Read the model definition and answer for the solid it produces. Units are mm, in the model's axes. Face numbers are marked on the shaded views. A direction names the side the tool comes from. Round coordinates to 2 decimals unless told otherwise and drop trailing zeros. Order: outer loops, then holes, each group sorted by start corner. A loop starts at its lowest first (then second) coordinate and runs counter-clockwise, first axis right, second up. Notation, with made-up numbers: (-16, -2) - (30, -2) arc R22 cw to (30, 5) - close; hole circle Ø4 at (7.25, 9). An arc over 180 degrees is marked (long way). Answer as a JSON object with one key per item and string values. Group by question number.
Q1. Given pin 1 Ø5 at (x, z) = (25.5, 93) entering from +Y; pin 2 Ø7.5 at (y, z) = (-12.5, 79) entering from -X; pin 3 Ø5.5 at (x, y) = (20, 34) entering from +Z; pin 4 Ø6.5 at (x, y) = (0, 17.5) entering from -Z (3 decimals), each flat-ended and moving along its own axis, determine where each tip first touches the part or whether it passes through.
Q2. Consider line 1 (Y direction, x = 0, z = -1); line 2 (Y direction, x = 0, z = 2); line 3 (Y direction, x = 20, z = 2). Determine where each line is inside the solid, lowest interval first.
Q3. A cutting plane is placed at A-A on y = -12.5. Count the separate pieces of the cut face and the enclosed holes in it, and give its area (3 significant figures).
Q4. A tool of negligible diameter and unlimited length cuts with its end or side. For the marked faces 5, 6, 7, 8 and 9, from which of +Z, -Z, +X, -X, +Y, -Y can it reach the whole face along a straight path? Write none if from no direction.
Q5. A cutting plane is placed at C-C on y = 32.5. Determine the outline of the cut face in (x, z).
Q6. The mould has two halves that part along X. Classify the marked faces 1, 2, 3 and 4: pulls with the +X half, pulls with the -X half, needs draft (parallel to the pull), parting line crosses it, or undercut.
Q7. A cutting plane is placed at B-B on x = -49. Determine the outline of the cut face in (y, z).
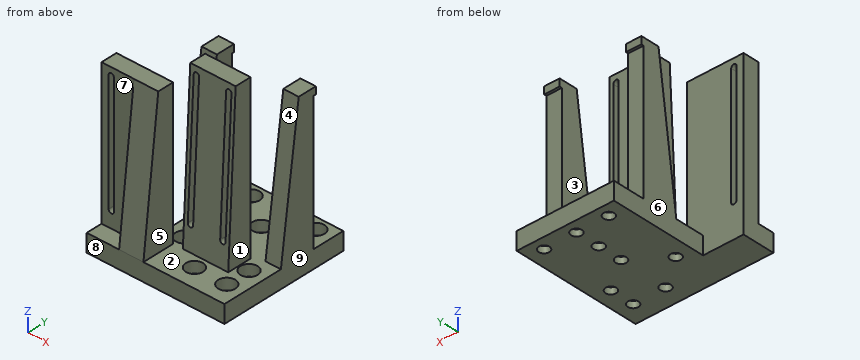
```python
from build123d import *

# Parameters (mm, degrees)
SKETCH1_W                 = 60
SKETCH1_H                 = 80
SKETCH1_R                 = 3.3
BOSS_EXTRUDE1_DEPTH       = 4
SKETCH3_W                 = 60
SKETCH3_H                 = 80
SKETCH3_R                 = 5.3
BOSS_EXTRUDE2_DEPTH       = 7
SKETCH4_W                 = 9.5
SKETCH4_H                 = 10
BOSS_EXTRUDE3_DEPTH       = 89
BOSS_EXTRUDE4_DEPTH       = 9.5
BOSS_EXTRUDE5_DEPTH       = 9.5
SKETCH7_W                 = 9.5
SKETCH7_H                 = 4.5
BOSS_EXTRUDE6_DEPTH       = 1.5
SKETCH9_W                 = 28
SKETCH9_H                 = 10
BOSS_EXTRUDE7_DEPTH       = 100
BOSS_EXTRUDE9_DEPTH       = 28
CUT_EXTRUDE1_DEPTH        = 18
BOSS_EXTRUDE10_DEPTH      = 25
BOSS_EXTRUDE10_DEPTH_BACK = 10
SKETCH13_W                = 100
SKETCH13_H                = 10
SKETCH14_W                = 11
SKETCH14_H                = 20
BOSS_EXTRUDE11_DEPTH      = 25
CUT_EXTRUDE2_DEPTH        = 10
BOSS_EXTRUDE12_DEPTH      = 15


with BuildPart() as part:
    # Sketch1 → Boss-Extrude1 (new body)
    with BuildSketch(Plane.XY):
        Rectangle(SKETCH1_W, SKETCH1_H)
        with Locations((-20, -12.5)):
            Circle(SKETCH1_R, mode=Mode.SUBTRACT)
        with Locations((20, -12.5)):
            Circle(SKETCH1_R, mode=Mode.SUBTRACT)
        with Locations((0, 17.5)):
            Circle(SKETCH1_R, mode=Mode.SUBTRACT)
        with Locations((0, 2.5)):
            Circle(SKETCH1_R, mode=Mode.SUBTRACT)
        with Locations((20, 32.5)):
            Circle(SKETCH1_R, mode=Mode.SUBTRACT)
        with Locations((0, 32.5)):
            Circle(SKETCH1_R, mode=Mode.SUBTRACT)
        with Locations((-20, 32.5)):
            Circle(SKETCH1_R, mode=Mode.SUBTRACT)
        with Locations((0, -27.5)):
            Circle(SKETCH1_R, mode=Mode.SUBTRACT)
        with Locations((20, -27.5)):
            Circle(SKETCH1_R, mode=Mode.SUBTRACT)
    extrude(amount=-BOSS_EXTRUDE1_DEPTH)

    # Sketch3 → Boss-Extrude2 (add)
    with BuildSketch(Plane.XY):
        Rectangle(SKETCH3_W, SKETCH3_H)
        with Locations((0, 17.5)):
            Circle(SKETCH3_R, mode=Mode.SUBTRACT)
        with Locations((-20, -12.5)):
            Circle(SKETCH3_R, mode=Mode.SUBTRACT)
        with Locations((20, -12.5)):
            Circle(SKETCH3_R, mode=Mode.SUBTRACT)
        with Locations((0, 2.5)):
            Circle(SKETCH3_R, mode=Mode.SUBTRACT)
        with Locations((-20, 32.5)):
            Circle(SKETCH3_R, mode=Mode.SUBTRACT)
        with Locations((0, 32.5)):
            Circle(SKETCH3_R, mode=Mode.SUBTRACT)
        with Locations((20, 32.5)):
            Circle(SKETCH3_R, mode=Mode.SUBTRACT)
        with Locations((0, -27.5)):
            Circle(SKETCH3_R, mode=Mode.SUBTRACT)
        with Locations((20, -27.5)):
            Circle(SKETCH3_R, mode=Mode.SUBTRACT)
    extrude(amount=BOSS_EXTRUDE2_DEPTH)

    # Sketch4 → Boss-Extrude3 (add)
    with BuildSketch(Plane.XY.offset(7)):
        with Locations((-25.25, 15)):
            Rectangle(SKETCH4_W, SKETCH4_H)
        with Locations((25.25, 15)):
            Rectangle(SKETCH4_W, SKETCH4_H)
    extrude(amount=BOSS_EXTRUDE3_DEPTH)

    # Sketch5 → Boss-Extrude4 (add)
    with BuildSketch(Plane(origin=(30, 0, 0), x_dir=(0, 0, -1), z_dir=(1, 0, 0))):
        Polygon((-96, 10), (-7, 10), (-7, -2), align=None)
    extrude(amount=-BOSS_EXTRUDE4_DEPTH)

    # Sketch6 → Boss-Extrude5 (add)
    with BuildSketch(Plane.ZY.offset(30)):
        Polygon((96, 10), (7, 10), (7, -2), align=None)
    extrude(amount=-BOSS_EXTRUDE5_DEPTH)

    # Sketch7 → Boss-Extrude6 (add)
    with BuildSketch(Plane(origin=(0, 20, 0), x_dir=(1, 0, 0), z_dir=(0, 1, 0))):
        with Locations((-25.25, -93.75)):
            Rectangle(SKETCH7_W, SKETCH7_H)
        with Locations((25.25, -93.75)):
            Rectangle(SKETCH7_W, SKETCH7_H)
    extrude(amount=BOSS_EXTRUDE6_DEPTH)

    # Sketch9 → Boss-Extrude7 (add)
    with BuildSketch(Plane.XY.offset(7)):
        with Locations((0, -10)):
            Rectangle(SKETCH9_W, SKETCH9_H)
    extrude(amount=BOSS_EXTRUDE7_DEPTH)

    # Sketch11 → Boss-Extrude9 (add)
    with BuildSketch(Plane.ZY.offset(14)):
        Polygon((107, -15), (7, -15), (7, -20), align=None)
    extrude(amount=-BOSS_EXTRUDE9_DEPTH)

    # Sketch12 → Cut-Extrude1 (cut)
    with BuildSketch(Plane(origin=(0, -5, 0), x_dir=(1, 0, 0), z_dir=(0, 1, 0))):
        with BuildLine():
            Line((-11.65, -22), (-11.65, -102))
            ThreePointArc((-11.65, -102), (-10, -103.65), (-8.35, -102))
            Line((-8.35, -102), (-8.35, -22))
            ThreePointArc((-8.35, -22), (-10, -20.35), (-11.65, -22))
        make_face()
        with BuildLine():
            Line((8.35, -22), (8.35, -102))
            ThreePointArc((8.35, -102), (10, -103.65), (11.65, -102))
            Line((11.65, -102), (11.65, -22))
            ThreePointArc((11.65, -22), (10, -20.35), (8.35, -22))
        make_face()
    extrude(amount=-CUT_EXTRUDE1_DEPTH, mode=Mode.SUBTRACT)



with BuildPart() as body_2:
    # Sketch13 → Boss-Extrude10 (new, two sides: drawn at the far end of the back side and taken through both)
    with BuildSketch(Plane.ZY.offset(30).offset(-BOSS_EXTRUDE10_DEPTH_BACK)):
        with Locations((46, -25)):
            Rectangle(SKETCH13_W, SKETCH13_H)
    extrude(amount=BOSS_EXTRUDE10_DEPTH + BOSS_EXTRUDE10_DEPTH_BACK)


with BuildPart() as part_1:
    add(part.part)

    add(body_2.part)  # Boss-Extrude11 merges body 2
    # Sketch14 → Boss-Extrude11 (add)
    with BuildSketch(Plane.ZY.offset(30)):
        with Locations((1.5, -30)):
            Rectangle(SKETCH14_W, SKETCH14_H)
    extrude(amount=BOSS_EXTRUDE11_DEPTH)

    # Sketch15 → Cut-Extrude2 (cut)
    with BuildSketch(Plane(origin=(0, -20, 0), x_dir=(1, 0, 0), z_dir=(0, 1, 0))):
        with BuildLine():
            Line((-50.65, -91), (-50.65, -17))
            ThreePointArc((-50.65, -17), (-48.959530594, -15.350496369), (-47.351985179, -17.080914463))
            Line((-47.351985179, -17.080914463), (-47.351985179, -91.080914463))
            ThreePointArc((-47.351985179, -91.080914463), (-49.040469406, -92.649503631), (-50.65, -91))
        make_face()
    extrude(amount=-CUT_EXTRUDE2_DEPTH, mode=Mode.SUBTRACT)

    # Sketch16 → Boss-Extrude12 (add)
    with BuildSketch(Plane(origin=(-20, 0, 0), x_dir=(0, 0, -1), z_dir=(1, 0, 0))):
        Polygon((-96, -30), (-7, -30), (-7, -40), align=None)
    extrude(amount=-BOSS_EXTRUDE12_DEPTH)


solid = part_1.part
```
Result set:
{
 "1": {"pin 1": "stops at y = 21.5", "pin 2": "stops at x = -14", "pin 3": "stops at z = 0", "pin 4": "passes through"},
 "2": {"line 1": "y = -40 to -30.8, -24.2 to -0.8, 5.8 to 14.2, 20.8 to 29.2, 35.8 to 40", "line 2": "y = -40 to -32.8, -22.2 to -2.8, 7.8 to 12.2, 22.8 to 27.2, 37.8 to 40", "line 3": "y = -40 to -32.8, -22.2 to -17.8, -7.2 to 27.2, 37.8 to 40"},
 "3": {"separate pieces": "3", "enclosed holes": "2", "area": "2,710 mm²"},
 "4": {"face 5": "+Z, +X, +Y, -Y", "face 6": "+Z, -Z, -X, +Y", "face 7": "+Z, -X, -Y", "face 8": "+Z, -Z, +X, -X, -Y", "face 9": "+Z, -Z, +X, +Y, -Y"},
 "5": {"outline": "(-30, -4) - (-23.3, -4) - (-23.3, 0) - (-25.3, 0) - (-25.3, 7) - (-30, 7) - close; (-16.7, -4) - (-3.3, -4) - (-3.3, 0) - (-5.3, 0) - (-5.3, 7) - (-14.7, 7) - (-14.7, 0) - (-16.7, 0) - close; (3.3, -4) - (16.7, -4) - (16.7, 0) - (14.7, 0) - (14.7, 7) - (5.3, 7) - (5.3, 0) - (3.3, 0) - close; (23.3, -4) - (30, -4) - (30, 7) - (25.3, 7) - (25.3, 0) - (23.3, 0) - close"},
 "6": {"face 1": "pulls with the +X half", "face 2": "undercut", "face 3": "undercut", "face 4": "needs draft"},
 "7": {"outline": "(-40, -4) - (-20, -4) - (-20, 15.35) - (-30, 15.35) - (-30, 7) - (-40, 7) - close; (-30, 92.65) - (-20, 92.65) - (-20, 96) - (-30, 96) - close"}
}
